from build123d import *

# Parameters (mm, degrees)
BOSS_EXTRUDE1_DEPTH = 57.15
CUT_EXTRUDE1_DEPTH  = 57.15
SKETCH3_R           = 2.032
CUT_EXTRUDE2_DEPTH  = 401.855538193


with BuildPart() as part:
    # Sketch1 → Boss-Extrude1 (new body)
    with BuildSketch(Plane(origin=(0, 0, 0), x_dir=(1, 0, 0), z_dir=(0, 1, 0))):
        Polygon((-152.4, 0), (152.4, 0), (152.4, -127), (63.5, -177.8), (63.5, -254), (-63.5, -254), (-63.5, -177.8), (-152.4, -127), align=None)
    extrude(amount=BOSS_EXTRUDE1_DEPTH)

    # Sketch2 → Cut-Extrude1 (cut)
    with BuildSketch(Plane(origin=(0, 57.15, 0), x_dir=(1, 0, 0), z_dir=(0, 1, 0))):
        Polygon((-139.7, -6.35), (139.7, -6.35), (139.7, -120.65), (57.15, -171.45), (57.15, -247.65), (-57.15, -247.65), (-57.15, -171.45), (-139.7, -120.65), align=None)
    extrude(amount=-CUT_EXTRUDE1_DEPTH, mode=Mode.SUBTRACT)

    # Sketch3 → Cut-Extrude2 (cut, through all)
    with BuildSketch(Plane(origin=(152.4, 0, 0), x_dir=(0, 0, -1), z_dir=(1, 0, 0))):
        with Locations((-57.15, 19.685)):
            Circle(SKETCH3_R)
    extrude(amount=-CUT_EXTRUDE2_DEPTH, mode=Mode.SUBTRACT)


solid = part.part
Could you check a few things on this model? Use its own coordinates, in mm. A direction names the side the tool comes from. Round coordinates to 2 decimals unless told otherwise and drop trailing zeros. Write each loop counter-clockwise with the first axis right and the second up, starting at its lowest first coordinate (ties: lowest second). Pieces come first, ordered by that corner, then holes. Notation, with made-up numbers: (10.5, 14.25) - (62.5, 14.25) arc R28 ccw to (62.5, 34.25) - close; hole circle Ø10 at (8, -31). An arc over 180 degrees is marked (long way). Put each result on its own line as item: value. Start each with the question number.
(1) I want a section at B-B, the plane x = -4. Please give me the cut outline in (y, z).
(2) Thinking about a two-plate mould opening in Z: for faces 1 (the flat face through (-152.4, 28, 64)), 2 (the flat face through (-57.15, 29, 210)), 3 (the flat face through (108.572, 28.175, 152.044)), which applies, released by +Z, released by -Z, zero draft, split by the parting line, or undercut?
(3) I want a section at A-A, the plane z = 40. Please give me the cut outline in (x, y), plus the area to 3 significant figures.
(4) I need wall thicknesses on probe 1 along Z at (x, y) = (-44.5, 21.5); probe 2 along X at (y, z) = (40, 184); probe 3 along Y at (x, z) = (143, 57). Which ranges of each line are inside material? Lowest first, please.
(5) Will these pins go through, and if not, where does the flat tip stop? pin 1 (17 mm diameter, centred on y = 37, z = 201.5, fed in from +X); pin 2 (3.5 mm diameter, centred on y = 19.685, z = 57.15, fed in from +X).
(6) I want a section at C-C, the plane y = 5. Please give me the cut outline in (x, z), plus the area to 3 significant figures.
(7) For faces 4 (the flat face through (1, 0, 4)), 5 (the flat face through (-63.5, 28, 216)), 6 (the flat face through (63.5, 28, 215)), 7 (the flat face through (99.003, 28.975, 145.694)), which set-ups out of +Z, -Z, +X, -X, +Y, -Y let a thin tool reach every point of the face, with its end or its side?
Here are the results:
1. outline: (0, 0) - (57.15, 0) - (57.15, 6.35) - (0, 6.35) - close; (0, 247.65) - (57.15, 247.65) - (57.15, 254) - (0, 254) - close
2. face 1: zero draft
2. face 2: undercut
2. face 3: released by +Z
3. outline: (-152.4, 0) - (-139.7, 0) - (-139.7, 57.15) - (-152.4, 57.15) - close; (139.7, 0) - (152.4, 0) - (152.4, 57.15) - (139.7, 57.15) - close
3. area: 1,450 mm^2
4. probe 1: z = 0 to 6.35, 247.65 to 254
4. probe 2: x = -63.5 to -57.15, 57.15 to 63.5
4. probe 3: y = 0 to 17.66, 21.71 to 57.15
5. pin 1: stops at x = 63.5
5. pin 2: passes through
6. outline: (-152.4, 0) - (152.4, 0) - (152.4, 127) - (63.5, 177.8) - (63.5, 254) - (-63.5, 254) - (-63.5, 177.8) - (-152.4, 127) - close; hole (-139.7, 6.35) - (139.7, 6.35) - (139.7, 120.65) - (57.15, 171.45) - (57.15, 247.65) - (-57.15, 247.65) - (-57.15, 171.45) - (-139.7, 120.65) - close
6. area: 8,710 mm^2
7. face 4: +Z, -Z, +X, -X, -Y
7. face 5: +Z, -X, +Y, -Y
7. face 6: +Z, +X, +Y, -Y
7. face 7: +Y, -Y
